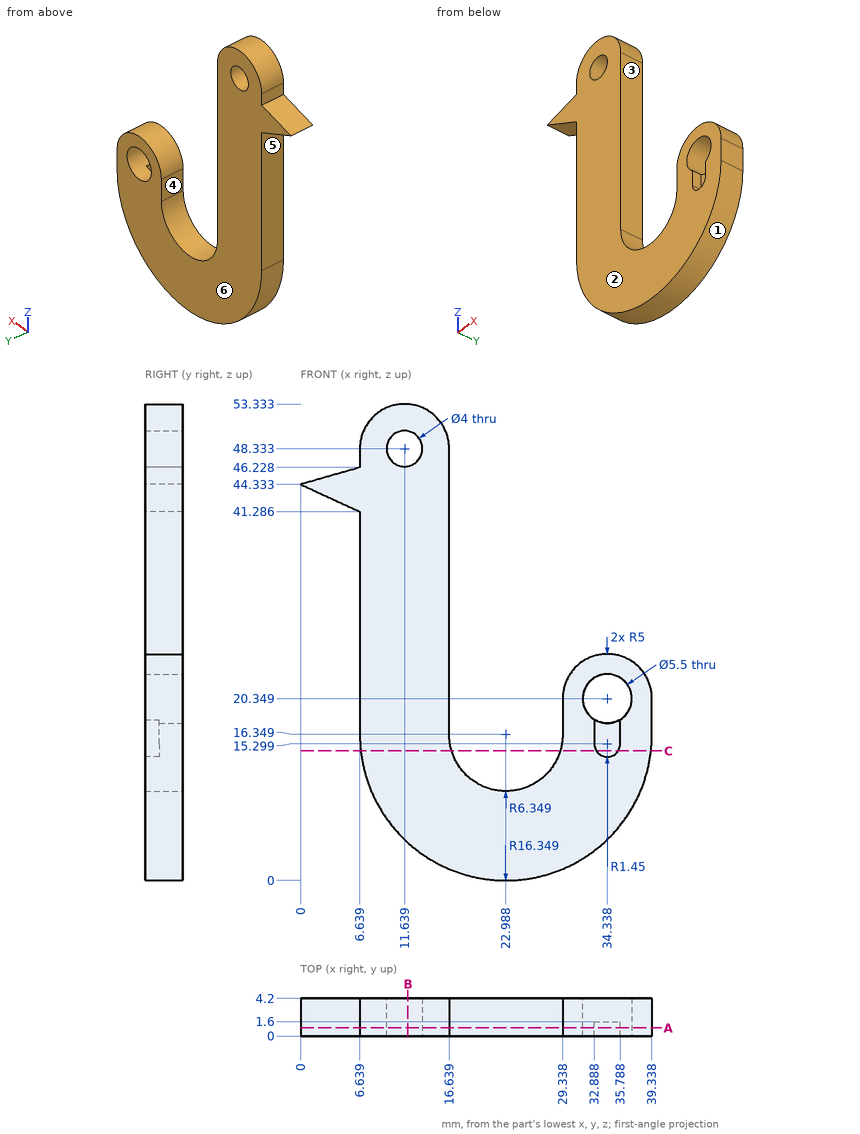
The figure shows three views and two pictorial views of one solid part (mm, origin at its lowest corner). Answer the questions. A direction names the side the tool comes from. Round coordinates to 2 decimals unless told otherwise and drop trailing zeros. Order: outer loops, then holes, each group sorted by start corner. A loop starts at its lowest first (then second) coordinate and runs counter-clockwise, first axis right, second up. Notation, with made-up numbers: M 3.25,62.25 L 41.25,62.25 A15 cw 41.25,73.25 Z; hole C 38.5,16.5 d3. An arc over 180 degrees is marked long. Put each result on its own line as item: value. Start each with the question number.
Q1. Section B-B, the plane x = 12 is taken. Write down the section's boundary in (y, z) (1 decimal).
Q2. Section C-C, the plane z = 14.5 is taken. Write down the section's boundary in (x, y) (1 decimal).
Q3. Flat-ended cylindrical pins translate along their axes: pin 1 (1.3 mm diameter, centred on y = 3, z = 29.5, fed in from -X); pin 2 (2 mm diameter, centred on y = 3.5, z = 8, fed in from -X). Find the tip coordinate at first contact, or state that the pin passes through.
Q4. Section A-A, the plane y = 0.9 is taken. Give the number of separate pieces and of enclosed holes in the cut face.
Q5. For a pull along X with two mould halves and no side action, classify the marked faces 1, 2 and 3 as pulls with the +X half, pulls with the -X half, needs draft (parallel to the pull), parting line crosses it, or undercut.
Q6. A tool of negligible diameter and unlimited length cuts with its end or side. For the marked faces 4, 5 and 6, from which of +Z, -Z, +X, -X, +Y, -Y can it reach the whole face along a straight path? Write none if from no direction.
Q7. Straight lines are drawn through the part: L1, parallel to X at y = 1.3, z = 20.5 (1 decimal); L2, parallel to X at y = 2.3, z = 21.5 (1 decimal); L3, parallel to X at y = 3.25, z = 28. For each, find the intervals that lie inside material, in ascending order. Write a range as [from, to].
Findings below:
1. outline: M 0,4.2 L 4.2,4.2 L 4.2,46.4 L 0,46.4 Z; M 0,50.3 L 4.2,50.3 L 4.2,53.3 L 0,53.3 Z
2. outline: M 6.7,0 L 16.9,0 L 16.9,4.2 L 6.7,4.2 Z; M 29.1,0 L 33.1,0 L 33.1,1.6 L 35.5,1.6 L 35.5,0 L 39.2,0 L 39.2,4.2 L 29.1,4.2 Z
3. pin 1: stops at x = 6.64
3. pin 2: stops at x = 8.38
4. separate pieces: 1
4. enclosed holes: 2
5. face 1: parting line crosses it
5. face 2: needs draft
5. face 3: undercut
6. face 4: +Z, +Y, -Y
6. face 5: -Z, -X, +Y, -Y
6. face 6: +Z, -Z, +X, -X, +Y
7. L1: x = [6.6, 16.6], [29.3, 31.6], [37.1, 39.3]
7. L2: x = [6.6, 16.6], [29.5, 31.8], [36.8, 39.2]
7. L3: x = [6.64, 16.64]
